Can you work these out from the model? Positions are in its coordinate system, mm. Face numbers are marked on the shaded views. A direction names the side the tool comes from. Coordinates: 2 decimals unless noted, no trailing zeros. Loops run counter-clockwise (first coordinate to the right, second up) from the corner with the lowest first, then second, coordinate; pieces in that order, holes last.
```python
from build123d import *

# Parameters (mm, degrees)
F0_W     = 1200
F0_H     = 700
F1_DEPTH = 300
F2_R     = 30.5098573856
F3_DEPTH = 50
F3_TAPER = -3
F5_DEPTH = 560


with BuildPart() as f1:
    # F0 (on Top) → F1 (new body)
    with BuildSketch(Plane.XY):
        Rectangle(F0_W, F0_H)
    extrude(amount=F1_DEPTH)

    # F2 (on face) → F3 (join)
    with BuildSketch(Plane(origin=(0, 0, 0), x_dir=(1, 0, 0), z_dir=(0, 0, -1))):
        with Locations((-532.1071147919, -296.6614961624)):
            Circle(F2_R)
        with Locations((532.1071147919, -296.6614961624)):
            Circle(F2_R)
        with Locations((532.1071147919, 296.6614961624)):
            Circle(F2_R)
        with Locations((-532.1071147919, 296.6614961624)):
            Circle(F2_R)
    extrude(amount=F3_DEPTH, taper=F3_TAPER)

    # F4 (on Right) → F5 (join, symmetric)
    with BuildSketch(Plane.YZ):
        Polygon((-305.8277244632, 230.5950983165), (-107.0006990349, 254.912089853), (-270.1073586941, 750), (-350, 750), align=None)
    extrude(amount=F5_DEPTH, both=True)


solid = f1.part
```
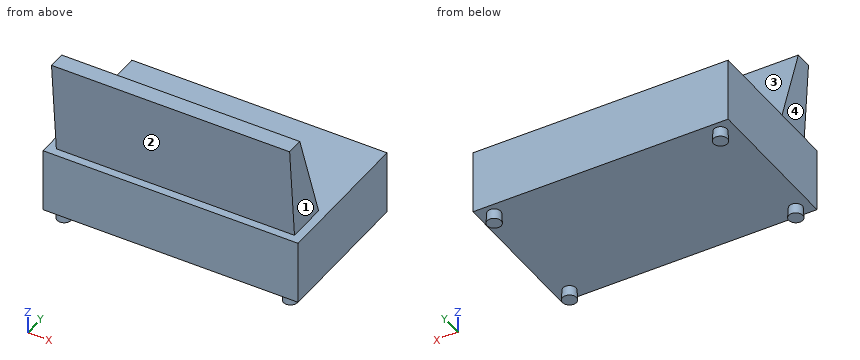
Item 1: Suppose I cut it at A-A, the plane x = -246. Please give me the cut outline in (y, z).
Results are:
outline: (-350, 0) - (350, 0) - (350, 300) - (-121.85, 300) - (-270.11, 750) - (-350, 750) - (-311.73, 300) - (-350, 300) - close
Item 2: On a 3-axis mill with a long thin cutter (end or side, diameter ignored), from which of +Z, -Z, +X, -X, +Y, -Y can I reach the whole of each face in a straight line? I mean the marked faces 1, 2, 3 and 4. Say none if no direction works.
Results are:
face 1: +Z, +X, +Y, -Y
face 2: +X, -X, -Y
face 3: +Z, +X, -X, +Y
face 4: +Z, -X, +Y, -Y
Item 3: Suppose I cut it at C-C, the plane z = 445. Please give me the cut outline in (x, y).
Results are:
outline: (-560, -324.06) - (560, -324.06) - (560, -169.63) - (-560, -169.63) - close
Item 4: Suppose I cut it at B-B, the plane y = -156. Please give me the cut outline in (x, z).
Results are:
outline: (-600, 0) - (600, 0) - (600, 300) - (560, 300) - (560, 403.64) - (-560, 403.64) - (-560, 300) - (-600, 300) - close
Item 5: I need wall thicknesses on line 1 along Z through (x, y) = (-340, 178.5); line 2 along X through (y, z) = (-187.5, 393); line 3 along Z through (x, y) = (-43, -299.5). Which ranges of each line are inside material? Lowest first, please.
Results are:
line 1: z = 0 to 300
line 2: x = -560 to 560
line 3: z = 0 to 750
Item 6: Suppose I cut it at D-D, the plane y = 39. Please give me the cut outline in (x, z), plus the area to 3 significant figures.
Results are:
outline: (-600, 0) - (600, 0) - (600, 300) - (-600, 300) - close
area: 360,000 mm2
Item 7: I'm going to push flat-ended pins straight in: P1, Ø10, axis at x = 344.5, z = 661, coming from the +Y side; P2, Ø1, axis at x = -30, y = -210.5, coming from the -Z side; P3, Ø8, axis at x = -375.5, z = 439, coming from the -Y side. Where does each tip first touch, or does it pass through?
Results are:
P1: stops at y = -239.14
P2: stops at z = 0
P3: stops at y = -323.89
